Autodesk Inventor part; units mm, degrees
ref_plane "YZ Plane" through (0, 0, 0) normal (1, 0, 0) x (0, 1, 0)
ref_plane "XZ Plane" through (0, 0, 0) normal (0, 1, 0) x (-1, 0, 0)
ref_plane "XY Plane" through (0, 0, 0) normal (0, 0, 1) x (1, 0, 0)
sketch "Sketch1" plane through (0, 0, 0) normal (0, 1, 0) x (-1, 0, 0)
  arc A0 (0, 150) -> (0, -150) centre (0, 0) ccw
  arc A1 (0, 130) -> (0, -130) centre (0, 0) ccw
  line L0 (0, -150) -> (0, 150)
  line L1 (150, 0) -> (-150, 0)
  circle A2 centre (0, 0) radius 141
  dimension "d0" = 300
  dimension "d1" = 260
  dimension "d9" = 282
revolve "Revolution1" add sketch "Sketch1" angle 180 about axis through (0, 0, -150) along (0, 0, -1) contours L0 A2 L1 A0 | L1 A2 L0 A0 | L0 A1 L1 A2 | L1 A1 L0 A2
sketch "Sketch6" plane through (0, 0, 0) normal (0, 1, 0) x (1, 0, 0)
  circle A0 centre (0, 0) radius 140
  circle A1 centre (0, 0) radius 128.5
  dimension "d19" = 280
  dimension "d20" = 257
extrude "Extrusion3" cut sketch "Sketch6" against normal blind 12.5
sketch "Sketch7" plane through (0, -12.5, 0) normal (0, 1, 0) x (1, 0, 0)
  line L0 (-5, 140.4975) -> (5, 140.4975)
  line L1 (5, 140.4975) -> (5, 128.8975)
  line L2 (5, 128.8975) -> (-5, 128.8975)
  line L3 (-5, 128.8975) -> (-5, 140.4975)
  circle A0 centre (0, 0) radius 129.3976
  arc A1 (-5, 129.301) -> (0, 129.3976) centre (0, 0) ccw
  circle A2 centre (0, 0) radius 140
  arc A3 (-5, 139.9107) -> (0, 140) centre (0, 0) ccw
  point P0 (5, 139.9107)
  point P1 (5, 129.301)
  dimension "d23" = 10
  dimension "d24" = 11.6
  dimension "d25" = 5
  dimension "d26" = 128.8975
extrude "Extrusion4" cut sketch "Sketch7" against normal blind 5 contours A2 L1 A0 L3 | A0 L1 L2 L3 picked at (4.4446, 132.8554) picked at (0, 129.0642)
pattern_circular "Circular Pattern1" count 8 over 360 about axis through (0, -10, 0) along (0, 1, 0) of "Extrusion4"
sketch "Sketch8" plane through (0, 0, 0) normal (0, 1, 0) x (1, 0, 0)
  circle A0 centre (0, 145) radius 1
  circle A1 centre (0, 0) radius 150
  dimension "d32" = 2
  dimension "d33" = 145
extrude "Extrusion5" cut sketch "Sketch8" against normal blind 7 contours A0
pattern_circular "Circular Pattern2" count 16 over 360 about axis through (0, -10, 0) along (0, 1, 0) of "Extrusion5"
properties part number "Bol" material "Glass"
Design review of the part built by this model. Coordinates are the model's own, in mm. Coordinates: 2 decimals unless noted, no trailing zeros. Loops run counter-clockwise (first coordinate to the right, second up) from the corner with the lowest first, then second, coordinate; pieces in that order, holes last. Notation, with made-up numbers: (-30.5, -36) -> (17.5, -36) arc R9 ccw to (17.5, -23) -> close; hole circle Ø11 at (-38.75, 78.25). An arc over 180 degrees is marked (long way). Use a Markdown table: item, result. Add a question column.
Item 1: Wall thickness on L1, parallel to X at y = -2, z = 0; L2, parallel to Z at x = 70.5, y = -66.5; L3, parallel to X at y = -50.5, z = 55: over which ranges is each line inside the solid? List them lowest first. Write a range as from..to.
Item 2: Clearance check with flat-ended pins moving along their axes: P1, Ø2, axis at x = 80.5, y = -20.5, coming from the +Z side; P2, Ø3, axis at y = -66.5, z = 113, coming from the +X side; P3, Ø12, axis at x = 2, y = -119.5, coming from the -Z side. State where each tip first meets the part, or that it passes through.
Item 3: We need section A-A, the plane z = -114.5. Write out the cut boundary in (x, y), and give its area (3 significant figures).
Item 4: We need section B-B, the plane y = -61. Write out the cut boundary in (x, z), and give its area (3 significant figures).
Item 5: The part is to be moulded in two halves that separate along Z. For faces 1 (the flat face through (-99.3, 0, -99.3)), 2 (the flat face through (-98.63, -14.96, 91.56)), say which applies: +Z half, -Z half, draft (parallel to the pull), parting line (faces both ways), or undercut.
Item 6: We need section C-C, the plane z = -22.5. Write out the cut boundary in (x, y).
Numbers:
| question | item | result |
|---|---|---|
| 1 | L1 | x = -149.99..-146, -144..-140, 140..144, 146..149.99 |
| 1 | L2 | z = -114.49..-86.65, 86.65..114.49 |
| 1 | L3 | x = -130.1..-106.42, 106.42..130.1 |
| 2 | P1 | stops at z = 125.56 |
| 2 | P2 | stops at x = 75.5 |
| 2 | P3 | stops at z = -98.05 |
| 3 | outline | (-96.9, 0) arc R96.9 ccw to (96.9, 0) -> (80.56, 0) -> (80.56, -12.5) -> (60.28, -12.5) arc R61.56 cw to (-60.28, -12.5) -> (-80.56, -12.5) -> (-80.56, 0) -> close |
| 3 | area | 8,310 mm^2 |
| 4 | outline | circle Ø274.07 at (0, 0); hole circle Ø229.6 at (0, 0) |
| 4 | area | 17,600 mm^2 |
| 5 | face 1 | draft |
| 5 | face 2 | undercut |
| 6 | outline | (-148.3, 0) arc R148.3 ccw to (148.3, 0) -> (138.18, 0) -> (138.18, -12.5) -> (127.43, -12.5) arc R128.04 cw to (-127.43, -12.5) -> (-138.18, -12.5) -> (-138.18, 0) -> close |
